from build123d import *

# Parameters (mm, degrees)
EXTRUDE_1_DEPTH     = 44
SKETCH_4_R          = 1.9
SKETCH_4_R_2        = 4.5
CUT_EXTRUDE_1_DEPTH = 52.536394907
CHAMFER_1_SIZE      = 10


with BuildPart() as part:
    # Эскиз2 → Вытянуть-Тонкостенный1 (new body)
    with BuildSketch(Plane.XY):
        Polygon((24, 0), (0, 0), (0, 14), (2, 14), (2, 2), (24, 2), align=None)
    extrude(amount=EXTRUDE_1_DEPTH)

    # Эскиз4 → Вырез-Вытянуть1 (cut, through all)
    with BuildSketch(Plane(origin=(0, 2, 0), x_dir=(-1, 0, 0), z_dir=(0, 1, 0))):
        with Locations(Location((-12.95, 14.5, 0), (0, 0, 90))):
            Circle(SKETCH_4_R)
        with Locations(Location((-12.95, 27, 0), (0, 0, 90))):
            Circle(SKETCH_4_R_2)
    extrude(amount=-CUT_EXTRUDE_1_DEPTH, mode=Mode.SUBTRACT)

    # Фаска1
    chamfer_1_edges = [part.edges().sort_by_distance(p)[0] for p in [
        (24, 1, 44),
    ]]
    chamfer(chamfer_1_edges, length=CHAMFER_1_SIZE)


solid = part.part
The model under review builds one solid part; all positions refer to its coordinate system, in mm. A direction names the side the tool comes from. Give positions to 0.01 mm unless a question says otherwise; leave off trailing zeros. Loops run counter-clockwise (first coordinate to the right, second up) from the corner with the lowest first, then second, coordinate; pieces in that order, holes last. Notation, with made-up numbers: (68.25, -27) -> (121.25, -27) arc R15 cw to (121.25, -10) -> close; hole circle Ø7 at (37.25, 78). An arc over 180 degrees is marked (long way). Put each result on its own line as item: value. Start each with the question number.
1. Wall thickness on probe 1 along X at (y, z) = (1.4, 27); probe 2 along X at (y, z) = (0.8, 14.5); probe 3 along Y at (x, z) = (3, 4): over which ranges is each line inside the solid? List them lowest first.
2. We need section C-C on x = 9.5. State the section outline as (y, z) points, then the cut area to 3 significant figures.
3. We need section A-A on x = 12.95. State the section outline as (y, z) points, then the cut area to 3 significant figures.
4. We need section D-D on z = 27. State the section outline as (x, y) points.
5. For faces 4 (the face through (1.8, 4.4, 44)), 5 (the face through (13, 2, 22)), list the 3-axis set-ups (+Z, -Z, +X, -X, +Y, -Y) from which the entire face can be reached by the end or side of a thin tool; tool diameter is ignored.
6. We need section B-B on z = 14.5. State the section outline as (x, y) points, then the cut area to 3 significant figures.
7. Clearance check with flat-ended pins moving along their axes: P1, Ø3.5, axis at x = 12.95, z = 14.5, coming from the -Y side; P2, Ø8, axis at x = 15.5, z = 39, coming from the +Y side; P3, Ø3.5, axis at y = 6, z = 24, coming from the +X side. State where each tip first meets the part, or that it passes through.
8. Mouldability with a two-part tool opening along X and no side actions: class faces 1 (the face through (2, 8, 22)), 2 (the face through (11.794, 1.014, 12.992)), 3 (the face through (9.4, 1.8, 0)) as released by +X, released by -X, zero draft, split by the parting line, or undercut.
Determined:
1. probe 1: 0 to 8.45, 17.45 to 24
1. probe 2: 0 to 11.05, 14.85 to 24
1. probe 3: 0 to 2
2. outline: (0, 0) -> (2, 0) -> (2, 24.11) -> (0, 24.11) -> close; (0, 29.89) -> (2, 29.89) -> (2, 44) -> (0, 44) -> close
2. area: 76.4 mm^2
3. outline: (0, 0) -> (2, 0) -> (2, 12.6) -> (0, 12.6) -> close; (0, 16.4) -> (2, 16.4) -> (2, 22.5) -> (0, 22.5) -> close; (0, 31.5) -> (2, 31.5) -> (2, 44) -> (0, 44) -> close
3. area: 62.4 mm^2
4. outline: (0, 0) -> (8.45, 0) -> (8.45, 2) -> (2, 2) -> (2, 14) -> (0, 14) -> close; (17.45, 0) -> (24, 0) -> (24, 2) -> (17.45, 2) -> close
5. face 4: +Z, +X, -X, +Y, -Y
5. face 5: +Z, -Z, +X, +Y
6. outline: (0, 0) -> (11.05, 0) -> (11.05, 2) -> (2, 2) -> (2, 14) -> (0, 14) -> close; (14.85, 0) -> (24, 0) -> (24, 2) -> (14.85, 2) -> close
6. area: 64.4 mm^2
7. P1: through
7. P2: y = 2
7. P3: x = 2
8. face 1: released by +X
8. face 2: undercut
8. face 3: zero draft
